Build history of the part. All positions in model axes, mm. A direction names the side the tool comes from. Give positions to 0.01 mm unless a question says otherwise; leave off trailing zeros. Loops run counter-clockwise (first coordinate to the right, second up) from the corner with the lowest first, then second, coordinate; pieces in that order, holes last. Notation, with made-up numbers: M 65,-31 L 95,-31 A14 cw 95,-4 Z; hole C -21.5,-15.75 d11. An arc over 180 degrees is marked long. Put each result on its own line as item: value.
```python
from build123d import *

# Parameters (mm, degrees)
ESBO_O1_W                  = 50
ESBO_O1_H                  = 100
RESSALTO_EXTRUS_O1_DEPTH   = 6
CORTE_EXTRUS_O1_DEPTH      = 105.394009728
CORTE_EXTRUS_O1_DEPTH_BACK = 105.394009728
ESBO_O2_R                  = 1.75
ESBO_O3_R                  = 1.75
CORTE_EXTRUS_O2_DEPTH      = 105.394009728
ESBO_O4_W                  = 10
ESBO_O4_H                  = 6
RESSALTO_EXTRUS_O2_DEPTH   = 6


with BuildPart() as part:
    # Esboço1 → Ressalto-extrusão1 (new body)
    with BuildSketch(Plane.XY):
        with Locations((-4.361697279, 50)):
            Rectangle(ESBO_O1_W, ESBO_O1_H)
    extrude(amount=RESSALTO_EXTRUS_O1_DEPTH)

    # Esboço2 → Corte-extrusão1 (cut, two sides: drawn at the far end of the back side and taken through both)
    with BuildSketch(Plane.XY.offset(6).offset(-CORTE_EXTRUS_O1_DEPTH_BACK)):
        with Locations((-24.361697279, 95)):
            Circle(ESBO_O2_R)
        with Locations((-24.361697279, 85)):
            Circle(ESBO_O2_R)
        with Locations((-24.361697279, 75)):
            Circle(ESBO_O2_R)
        with Locations((-24.361697279, 65)):
            Circle(ESBO_O2_R)
        with Locations((-24.361697279, 55)):
            Circle(ESBO_O2_R)
        with Locations((-24.361697279, 45)):
            Circle(ESBO_O2_R)
        with Locations((-24.361697279, 35)):
            Circle(ESBO_O2_R)
        with Locations((-24.361697279, 25)):
            Circle(ESBO_O2_R)
        with Locations((-24.361697279, 15)):
            Circle(ESBO_O2_R)
        with Locations((-24.361697279, 5)):
            Circle(ESBO_O2_R)
        with Locations((15.638302721, 95)):
            Circle(ESBO_O2_R)
        with Locations((15.638302721, 85)):
            Circle(ESBO_O2_R)
        with Locations((15.638302721, 75)):
            Circle(ESBO_O2_R)
        with Locations((15.638302721, 65)):
            Circle(ESBO_O2_R)
        with Locations((15.638302721, 55)):
            Circle(ESBO_O2_R)
        with Locations((15.638302721, 45)):
            Circle(ESBO_O2_R)
        with Locations((15.638302721, 35)):
            Circle(ESBO_O2_R)
        with Locations((15.638302721, 25)):
            Circle(ESBO_O2_R)
        with Locations((15.638302721, 15)):
            Circle(ESBO_O2_R)
        with Locations((15.638302721, 5)):
            Circle(ESBO_O2_R)
    extrude(amount=CORTE_EXTRUS_O1_DEPTH + CORTE_EXTRUS_O1_DEPTH_BACK, mode=Mode.SUBTRACT)

    # Esboço3 → Corte-extrusão2 (cut, through all)
    with BuildSketch(Plane.XY.offset(6)):
        with Locations((-4.361697279, 80)):
            Circle(ESBO_O3_R)
        with Locations((-4.361697279, 60)):
            Circle(ESBO_O3_R)
        with Locations((-4.361697279, 40)):
            Circle(ESBO_O3_R)
        with Locations((-4.361697279, 20)):
            Circle(ESBO_O3_R)
    extrude(amount=-CORTE_EXTRUS_O2_DEPTH, mode=Mode.SUBTRACT)

    # Esboço4 → Ressalto-extrusão2 (add)
    with BuildSketch(Plane(origin=(0, 0, 0), x_dir=(-1, 0, 0), z_dir=(0, -1, 0))):
        with Locations((4.361697279, -3)):
            Rectangle(ESBO_O4_W, ESBO_O4_H)
    extrude(amount=RESSALTO_EXTRUS_O2_DEPTH)


solid = part.part
```
Q1. Slice it at D-D (x = 5). List the corners of the cut face in (y, z).
Here are the results:
outline: M 0,0 L 100,0 L 100,6 L 0,6 Z
Q2. Drop flat-ended pins along their axis: pin 1 Ø4 at (x, y) = (-24.36, 75) entering from -Z; pin 2 Ø1.8 at (y, z) = (-3, 2.5) entering from +X. Give the stop position or say it passes through.
Here are the results:
pin 1: z = 0
pin 2: x = 0.64
Q3. Slice it at C-C (y = 15). List the corners of the cut face in (x, z), and give its area (3 significant figures).
Here are the results:
outline: M -29.36,0 L -26.11,0 L -26.11,6 L -29.36,6 Z; M -22.61,0 L 13.89,0 L 13.89,6 L -22.61,6 Z; M 17.39,0 L 20.64,0 L 20.64,6 L 17.39,6 Z
area: 258 mm²
Q4. Tool access for faces 1 (the flat face through (0.638, -3, 3)), 2 (the cylindrical face through (-23.55, 43.45, 2.96)): list every direction of +Z, -Z, +X, -X, +Y, -Y with a clear straight run to the whole face (end or side of a thin tool).
Here are the results:
face 1: +Z, -Z, +X, -Y
face 2: +Z, -Z
Q5. Slice it at B-B (z = 3.55). State how many separate pieces and enclosed holes the cut face has, and give its area (3 significant figures).
Here are the results:
separate pieces: 1
enclosed holes: 24
area: 4,830 mm²
Q6. Probe line 1 (Y direction, x = -4.5, z = 3.7); line 2 (X direction, y = 85, z = 4); line 3 (X direction, y = 44, z = 4.45). List the from-to ranges inside material, lowest first. Write a range as from..to.
Here are the results:
line 1: -6..18.26, 21.74..38.26, 41.74..58.26, 61.74..78.26, 81.74..100
line 2: -29.36..-26.11, -22.61..13.89, 17.39..20.64
line 3: -29.36..-25.8, -22.93..14.2, 17.07..20.64
Q7. Mould opens along Y. For faces 3 (the flat face through (-29.362, 49, 3)), 4 (the cylindrical face through (-22.745, 34.33, 2.958)) say: pulls with the +Y half, pulls with the -Y half, needs draft (parallel to the pull), parting line crosses it, or undercut.
Here are the results:
face 3: needs draft
face 4: undercut
Q8. Slice it at A-A (y = 40). List the corners of the cut face in (x, z), and give its area (3 significant figures).
Here are the results:
outline: M -29.36,0 L -6.11,0 L -6.11,6 L -29.36,6 Z; M -2.61,0 L 20.64,0 L 20.64,6 L -2.61,6 Z
area: 279 mm²
